Design review of the part built by this model. Coordinates are the model's own, in mm. Face numbers are marked on the shaded views. A direction names the side the tool comes from. Round coordinates to 2 decimals unless told otherwise and drop trailing zeros. Order: outer loops, then holes, each group sorted by start corner. A loop starts at its lowest first (then second) coordinate and runs counter-clockwise, first axis right, second up. Notation, with made-up numbers: (-12.5, -19) - (4.5, -19) arc R15 cw to (4.5, -4) - close; hole circle Ø11 at (72, 64). An arc over 180 degrees is marked (long way). Write item = value, one per line.
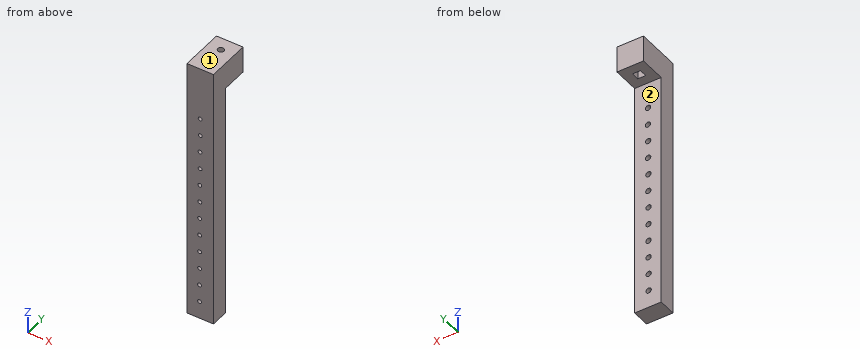
from build123d import *

# Parameters (mm, degrees)
SKETCH001_W      = 9
SKETCH001_H      = 9
PAD001_DEPTH     = 13
SKETCH002_R      = 3.5
PAD002_DEPTH     = 37
SKETCH_W         = 30
SKETCH_H         = 30
PAD_DEPTH        = 30
SKETCH003_W      = 30
SKETCH003_H      = 300
PAD003_DEPTH     = 20
HOLE_D           = 4.4
HOLE_DEPTH       = 25
HOLE_CBORE_D     = 6
HOLE_CBORE_DEPTH = 5


with BuildPart() as body001:
    # Sketch001 (on Face1 of CopyPad) → Pad001 (new body)
    with BuildSketch(Plane(origin=(0, 0, 0), x_dir=(1, 0, 0), z_dir=(0, 0, -1))):
        with Locations((15, -15)):
            Rectangle(SKETCH001_W, SKETCH001_H)
    extrude(amount=-PAD001_DEPTH)


with BuildPart() as body002:
    # Sketch002 (on Face1 of CopyPad001) → Pad002 (new body)
    with BuildSketch(Plane.XY.offset(50)):
        with Locations((15, 15)):
            Circle(SKETCH002_R)
    extrude(amount=-PAD002_DEPTH)


with BuildPart() as body:
    # Sketch → Pad (new body)
    with BuildSketch(Plane.XY):
        with Locations((15, 15)):
            Rectangle(SKETCH_W, SKETCH_H)
    extrude(amount=PAD_DEPTH)

    # Boolean: cut Body001
    add(body001.part, mode=Mode.SUBTRACT)

    # Boolean001: cut Body002
    add(body002.part, mode=Mode.SUBTRACT)


with BuildPart() as body003:
    # Sketch003 (on Face1 of CopyBoolean001) → Pad003 (new body)
    with BuildSketch(Plane.XZ):
        with Locations((15, -120)):
            Rectangle(SKETCH003_W, SKETCH003_H)
    extrude(amount=PAD003_DEPTH)

    # Hole
    with Locations(Plane(origin=(0, 0, 0), x_dir=(-1, 0, 0), z_dir=(0, 1, 0))):
        with Locations((-15, -50), (-14.956786, -30), (-14.77817, -90), (-14.734956, -70), (-14.559065, -130), (-14.515851, -110), (-14.337235, -170), (-14.294021, -150), (-14.335851, -210), (-14.292637, -190), (-14.231105, -250), (-14.187891, -230)):
            CounterBoreHole(HOLE_D / 2, HOLE_CBORE_D / 2, HOLE_CBORE_DEPTH, depth=HOLE_DEPTH)

    # Boolean002: union Body
    add(body.part)


solid = body003.part
1) We need section D-D on y = 25. Write out the cut boundary in (x, z), and give its area (3 significant figures).
Findings:
outline = (0, 0) - (30, 0) - (30, 30) - (0, 30) - close
area = 900 mm^2
2) We need section B-B on x = 4. Write out the cut boundary in (y, z).
Findings:
outline = (-20, -270) - (0, -270) - (0, 0) - (30, 0) - (30, 30) - (-20, 30) - close
3) To check wall thickness, follow L1, parallel to X at y = -11, z = -250; L2, parallel to Y at x = 21, z = -70.5; L3, parallel to Z at x = 12.25, y = 4. State the ranges of each line that lie inside material, in increasing order. Write a range as from..to.
Findings:
L1 = 0..12.03, 16.43..30
L2 = -20..0
L3 = 0..30
4) Clearance check with flat-ended pins moving along their axes: pin 1 Ø3 at (x, z) = (15, -211) entering from +Y; pin 2 Ø7 at (x, z) = (14.78, -90) entering from +Y; pin 3 Ø6 at (x, y) = (25.5, 12) entering from -Z; pin 4 Ø10 at (y, z) = (-9.5, -116) entering from -X. State where each tip first meets the part, or that it passes through.
Findings:
pin_1 = -5
pin_2 = 0
pin_3 = 0
pin_4 = 0
5) We need section C-C on z = -103. Write out the cut boundary in (x, y), and give its area (3 significant figures).
Findings:
outline = (0, -20) - (30, -20) - (30, 0) - (0, 0) - close
area = 600 mm^2
6) We need section A-A on y = -11.5. Give the number of separate pieces and of enclosed holes in the cut face, and give its area (3 significant figures).
Findings:
separate_pieces = 1
enclosed_holes = 12
area = 8,820 mm^2
7) For the marked faces 1 and 2, list the 3-axis set-ups (+Z, -Z, +X, -X, +Y, -Y) from which the entire face can be reached by the end or side of a thin tool; tool diameter is ignored.
Findings:
face_1 = +Z, +X, -X, +Y, -Y
face_2 = -Z, +X, -X, +Y
